from build123d import *

# Parameters (mm, degrees)
SKETCH1_W               = 12.7
SKETCH1_H               = 12.7
SKETCH1_W_2             = 9.525
SKETCH1_H_2             = 9.525
EXTRUDE_THIN1_DEPTH     = 508
SKETCH2_R               = 3.96875
CUT_EXTRUDE1_DEPTH      = 1.5875
SKETCH3_R               = 2.4765
CUT_EXTRUDE2_DEPTH      = 1
CUT_EXTRUDE2_DEPTH_BACK = 13.7
CUT_EXTRUDE3_REACH      = 14.7
SKETCH4_R               = 0.889
CUT_EXTRUDE4_REACH      = 14.7
SKETCH5_W               = 6.35
SKETCH5_H               = 9.525


with BuildPart() as part:
    # Sketch1 → Extrude-Thin1 (new body)
    with BuildSketch(Plane(origin=(0, 0, 0), x_dir=(1, 0, 0), z_dir=(0, 1, 0))):
        Rectangle(SKETCH1_W, SKETCH1_H)
        Rectangle(SKETCH1_W_2, SKETCH1_H_2, mode=Mode.SUBTRACT)
    extrude(amount=EXTRUDE_THIN1_DEPTH)

    # Sketch2 → Cut-Extrude1 (cut)
    with BuildSketch(Plane.XY.offset(6.35)):
        with Locations((0, 8.9123012)):
            Circle(SKETCH2_R)
    extrude(amount=-CUT_EXTRUDE1_DEPTH, mode=Mode.SUBTRACT)

    # Sketch3 → Cut-Extrude2 (cut, two sides)
    with BuildSketch(Plane.XY.offset(6.35)) as cut_extrude2_sk:
        with Locations((0, 501.65)):
            Circle(SKETCH3_R)
    extrude(amount=CUT_EXTRUDE2_DEPTH, mode=Mode.SUBTRACT)
    extrude(cut_extrude2_sk.sketch, amount=-CUT_EXTRUDE2_DEPTH_BACK, mode=Mode.SUBTRACT)

    # Sketch4 → Cut-Extrude3 (cut, up to next)
    with BuildSketch(Plane(origin=(6.35, 0, 0), x_dir=(0, 0, -1), z_dir=(1, 0, 0)), mode=Mode.PRIVATE) as cut_extrude3_sk1:
        with Locations((0, 9.525)):
            Circle(SKETCH4_R)
    cut_extrude3_tool1 = extrude(cut_extrude3_sk1.sketch, amount=-CUT_EXTRUDE3_REACH, mode=Mode.PRIVATE) & part.part
    add(cut_extrude3_tool1.solids().sort_by_distance((6.35, 9.525, 0))[0], mode=Mode.SUBTRACT)

    # Sketch5 → Cut-Extrude4 (cut, up to next)
    with BuildSketch(Plane.ZY.offset(6.35), mode=Mode.PRIVATE) as cut_extrude4_sk1:
        with Locations((0, 4.7625)):
            Rectangle(SKETCH5_W, SKETCH5_H)
    cut_extrude4_tool1 = extrude(cut_extrude4_sk1.sketch, amount=-CUT_EXTRUDE4_REACH, mode=Mode.PRIVATE) & part.part
    add(cut_extrude4_tool1.solids().sort_by_distance((-6.35, 4.7625, 0))[0], mode=Mode.SUBTRACT)


solid = part.part
The listing builds one solid part. Answer for the finished solid, in the listing's coordinates (mm). A direction names the side the tool comes from. Round coordinates to 2 decimals unless told otherwise and drop trailing zeros. Order: outer loops, then holes, each group sorted by start corner. A loop starts at its lowest first (then second) coordinate and runs counter-clockwise, first axis right, second up. Notation, with made-up numbers: M 19.5,2 L 76.5,2 A34 cw 76.5,39 Z; hole C 76.5,10 d2. An arc over 180 degrees is marked long. Answer in a Markdown table with one row per item. Add a question column.
1) Flat-ended cylindrical pins translate along their axes: pin 1 Ø4.5 at (x, y) = (0, 501.65) entering from +Z; pin 2 Ø1.7 at (x, z) = (-5.5, 1.5) entering from -Y (3 decimals); pin 3 Ø6.5 at (x, y) = (0, 8.91) entering from +Z; pin 4 Ø1.6 at (y, z) = (9.525, 0) entering from +X. Find the tip coordinate at first contact, or state that the pin passes through.
2) Which of the six approach directions +Z, -Z, +X, -X, +Y, -Y give full straight-line access (tool end or side, diameter ignored) to faces 1 (the face through (-4.762, 250, 0)), 2 (the face through (0, 250, -6.35))?
3) Determine the mould class of faces 3 (the face through (5, 0, 0)), 4 (the face through (6, 508, 0)), 5 (the face through (-0.517, 12.847, 5.567)), 6 (the face through (6.35, 250, 0)) for opening direction Y: pulls with the +Y half, pulls with the -Y half, needs draft (parallel to the pull), parting line crosses it, or undercut.
4) The part is cut by section A-A on y = 476. Determine the outline of the cut face in (x, z).
5) Consider line 1 along X through (y, z) = (208.5, -3.5); line 2 along X through (y, z) = (501.65, -5.25). Determine where each line is inside the solid, lowest interval first. Write a range as from..to.
6) The part is cut by section B-B on x = 0. Determine the outline of the cut face in (y, z).
Findings below:
| question | item | result |
|---|---|---|
| 1 | pin 1 | passes through |
| 1 | pin 2 | stops at y = 9.525 |
| 1 | pin 3 | stops at z = -4.76 |
| 1 | pin 4 | stops at x = -4.76 |
| 2 | face 1 | +Y, -Y |
| 2 | face 2 | -Z, +X, -X, +Y, -Y |
| 3 | face 3 | pulls with the -Y half |
| 3 | face 4 | pulls with the +Y half |
| 3 | face 5 | undercut |
| 3 | face 6 | needs draft |
| 4 | outline | M -6.35,-6.35 L 6.35,-6.35 L 6.35,6.35 L -6.35,6.35 Z; hole M -4.76,-4.76 L 4.76,-4.76 L 4.76,4.76 L -4.76,4.76 Z |
| 5 | line 1 | x = -6.35..-4.76, 4.76..6.35 |
| 5 | line 2 | x = -6.35..-2.48, 2.48..6.35 |
| 6 | outline | M 0,-6.35 L 499.17,-6.35 L 499.17,-4.76 L 0,-4.76 Z; M 0,4.76 L 4.94,4.76 L 4.94,6.35 L 0,6.35 Z; M 12.88,4.76 L 499.17,4.76 L 499.17,6.35 L 12.88,6.35 Z; M 504.13,-6.35 L 508,-6.35 L 508,-4.76 L 504.13,-4.76 Z; M 504.13,4.76 L 508,4.76 L 508,6.35 L 504.13,6.35 Z |
